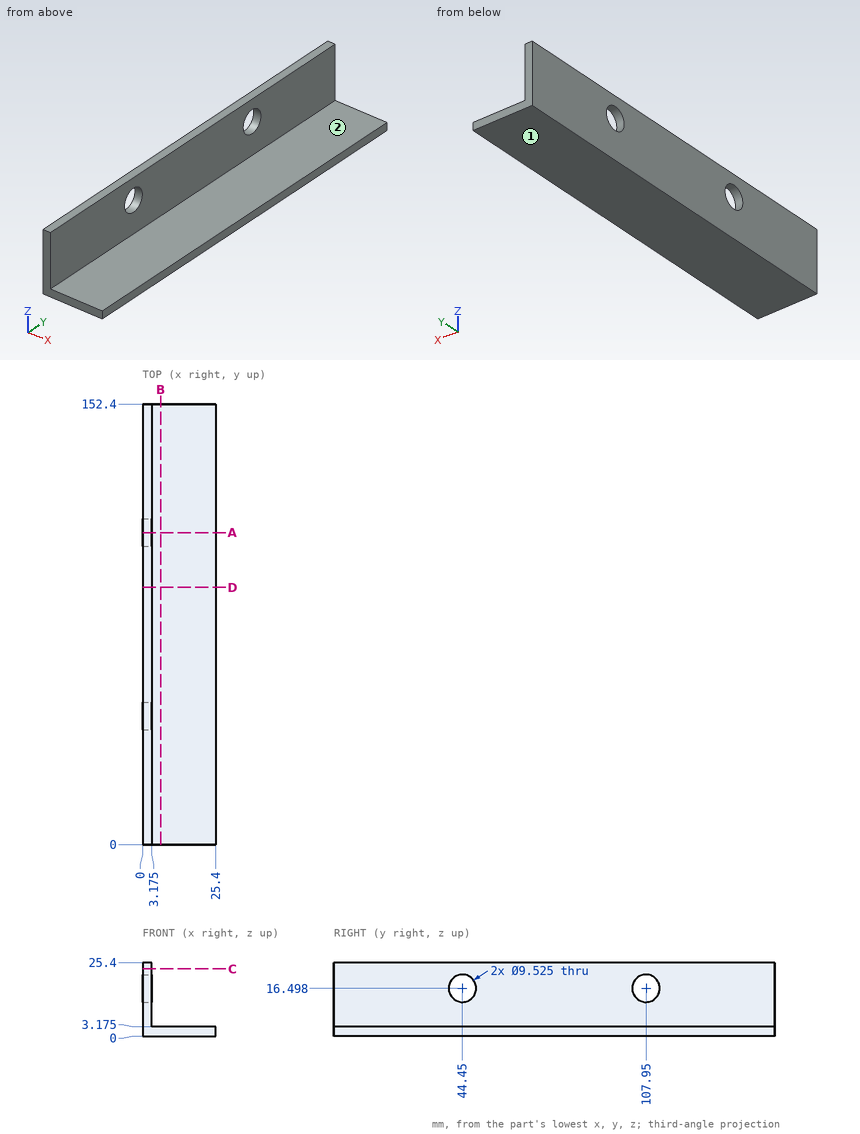
Study the drawing (mm; zero at the part's minimum x, y, z) and answer. A direction names the side the tool comes from. Coordinates: 2 decimals unless noted, no trailing zeros. Loops run counter-clockwise (first coordinate to the right, second up) from the corner with the lowest first, then second, coordinate; pieces in that order, holes last. Notation, with made-up numbers: M 47.5,43.5 L 70.5,43.5 A27 ccw 70.5,64.5 Z; hole C 68.25,12 d10. An arc over 180 degrees is marked long. Answer as a JSON object with one key per item and string values. Group by question number.
Item 1: Section A-A (y = 107.95) is taken. Write down the section's boundary in (x, z) (1 decimal).
Item 2: Consider L1, parallel to Y at x = 2, z = 16.25; L2, parallel to Z at x = 1.4, y = 44.45; L3, parallel to X at y = 92.5, z = 14 (3 decimals). Determine where each line is inside the solid, lowest interval first.
Item 3: Section D-D (y = 89) is taken. Write down the section's boundary in (x, z) (3 decimals).
Item 4: Section C-C (z = 23.25) is taken. Write down the section's boundary in (x, y) (3 decimals), and give its area (3 significant figures).
Item 5: Section B-B (x = 6.25) is taken. Write down the section's boundary in (y, z) (3 decimals).
Item 6: Which of the six approach directions +Z, -Z, +X, -X, +Y, -Y give full straight-line access (tool end or side, diameter ignored) to the marked faces 1 and 2?
Item 7: Each of these flat-tipped pins is pushed along its axis until it touches: P1, Ø10, axis at x = 14, y = 113.5, coming from the +Z side (3 decimals); P2, Ø1.5, axis at x = 19.5, z = 5, coming from the +Y side; P3, Ø8, axis at y = 31, z = 9, coming from the +X side (3 decimals). Where does it stop, or does it pass through?
Solved:
{
 "1": {"outline": "M 0,0 L 25.4,0 L 25.4,3.2 L 3.2,3.2 L 3.2,11.7 L 0,11.7 Z; M 0,21.3 L 3.2,21.3 L 3.2,25.4 L 0,25.4 Z"},
 "2": {"L1": "y = 0 to 39.69, 49.21 to 103.19, 112.71 to 152.4", "L2": "z = 0 to 11.74, 21.26 to 25.4", "L3": "x = 0 to 3.175"},
 "3": {"outline": "M 0,0 L 25.4,0 L 25.4,3.175 L 3.175,3.175 L 3.175,25.4 L 0,25.4 Z"},
 "4": {"outline": "M 0,0 L 3.175,0 L 3.175,152.4 L 0,152.4 Z", "area": "484 mm2"},
 "5": {"outline": "M 0,0 L 152.4,0 L 152.4,3.175 L 0,3.175 Z"},
 "6": {"face 1": "-Z, +X, -X, +Y, -Y", "face 2": "+Z, +X, +Y, -Y"},
 "7": {"P1": "stops at z = 3.175", "P2": "passes through", "P3": "stops at x = 3.175"}
}
